Work out the finished part from the listing and answer in its coordinate system (mm). Face numbers are marked on the shaded views. A direction names the side the tool comes from. Round coordinates to 2 decimals unless told otherwise and drop trailing zeros. Loops run counter-clockwise (first coordinate to the right, second up) from the corner with the lowest first, then second, coordinate; pieces in that order, holes last.
```python
from build123d import *

# Parameters (mm, degrees)
SKETCH_W             = 28
SKETCH_H             = 22
PAD002_DEPTH         = 5
POCKET001_DEPTH      = 0.8
SKETCH002_W          = 0.6
SKETCH002_H          = 23
POCKET_DEPTH         = 4
LINEARPATTERN_COUNT  = 11
LINEARPATTERN_PITCH  = 1.9
POCKET002_DEPTH      = 3.5
SKETCH006_W          = 28
SKETCH006_H          = 22
POCKET005_DEPTH      = 1
POCKET005_DEPTH_BACK = 1
PAD_DEPTH            = 2


with BuildPart() as part:
    # Sketch → Pad002 (new body)
    with BuildSketch(Plane.XY):
        with Locations((15, 12)):
            Rectangle(SKETCH_W, SKETCH_H)
    extrude(amount=PAD002_DEPTH)

    # Sketch001 → Pocket001 (cut)
    with BuildSketch(Plane.XY):
        with BuildLine():
            ThreePointArc((17.967868, 19.714572), (14.962963, 20.499886), (11.967982, 19.677535))
            Line((11.967982, 19.677535), (4.036475, 13.531422))
            ThreePointArc((4.036475, 13.531422), (3.750333, 12.536475), (4, 11.531754))
            Line((4, 11.531754), (12.33, 4.876817))
            ThreePointArc((12.33, 4.876817), (15.374304, 4.261687), (18.318313, 5.25112))
            Line((18.318313, 5.25112), (26, 11.531754))
            ThreePointArc((26, 11.531754), (26.249667, 12.536475), (25.963525, 13.531422))
            Line((25.963525, 13.531422), (17.967868, 19.714572))
        make_face()
    extrude(amount=POCKET001_DEPTH, mode=Mode.SUBTRACT)

    # Sketch002 → Pocket (cut)
    with BuildSketch(Plane.XY):
        with Locations((6.3, 11.5)):
            Rectangle(SKETCH002_W, SKETCH002_H)
    pocket = extrude(amount=POCKET_DEPTH, mode=Mode.SUBTRACT)

    # LinearPattern: Pocket ×11
    with Locations(*[(i * LINEARPATTERN_PITCH, 0, 0) for i in range(1, LINEARPATTERN_COUNT)]):
        add(pocket, mode=Mode.SUBTRACT)

    # Sketch003 → Pocket002 (cut)
    with BuildSketch(Plane(origin=(0.5, 0, 4), x_dir=(0.707107, 0, -0.707107), z_dir=(0.707107, 0, 0.707107))):
        with BuildLine():
            ThreePointArc((17.966363, 19.215428), (14.961232, 19.999875), (11.966488, 19.17666))
            Line((11.966488, 19.17666), (4.036475, 13.531422))
            ThreePointArc((4.036475, 13.531422), (3.750333, 12.536475), (4, 11.531754))
            Line((4, 11.531754), (12.33, 5.376817))
            ThreePointArc((12.33, 5.376817), (15.374304, 4.761687), (18.318313, 5.75112))
            Line((18.318313, 5.75112), (26, 11.531754))
            ThreePointArc((26, 11.531754), (26.249667, 12.536475), (25.963525, 13.531422))
            Line((25.963525, 13.531422), (17.966363, 19.215428))
        make_face()
    extrude(amount=POCKET002_DEPTH, mode=Mode.SUBTRACT)

    # Sketch006 → Pocket005 (cut, two sides)
    with BuildSketch(Plane.XY.offset(5)) as pocket005_sk:
        with Locations((15, 12)):
            Rectangle(SKETCH006_W, SKETCH006_H)
        with BuildLine():
            ThreePointArc((17.966363, 19.215428), (14.961232, 19.999875), (11.966488, 19.17666))
            Line((11.966488, 19.17666), (4.036475, 13.531422))
            ThreePointArc((4.036475, 13.531422), (3.750333, 12.536475), (4, 11.531754))
            Line((4, 11.531754), (12.33, 5.376817))
            ThreePointArc((12.33, 5.376817), (15.374304, 4.761687), (18.318313, 5.75112))
            Line((18.318313, 5.75112), (26, 11.531754))
            ThreePointArc((26, 11.531754), (26.249667, 12.536475), (25.963525, 13.531422))
            Line((25.963525, 13.531422), (17.966363, 19.215428))
        make_face(mode=Mode.SUBTRACT)
    extrude(amount=-POCKET005_DEPTH, mode=Mode.SUBTRACT)
    extrude(pocket005_sk.sketch, amount=POCKET005_DEPTH_BACK, mode=Mode.SUBTRACT)

    # Sketch004 → Pad (join)
    with BuildSketch(Plane.XY.offset(5)):
        Polygon((5, 19.805), (25, 19.805), (25, 15), (30, 15), (30, 10), (25, 10), (25, 4.805), (5, 4.805), (5, 10), (0, 10), (0, 15), (5, 15), align=None)
    extrude(amount=PAD_DEPTH)


solid = part.part
```
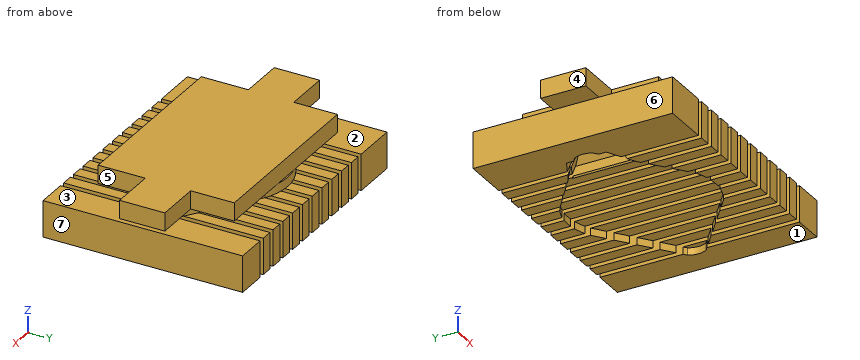
1. Find section A-A (x = 27). Write down the section's boundary in (y, z), then the cut area to 3 significant figures.
Answer key:
outline: (1, 0) - (23, 0) - (23, 4) - (1, 4) - close; (10, 5) - (15, 5) - (15, 7) - (10, 7) - close
area: 98.0 mm2
2. Find section D-D (x = 7). Write down the section's boundary in (y, z) (3 decimals), then the cut area to 3 significant figures.
Answer key:
outline: (1, 0) - (9.001, 0) - (9.135, 0.256) - (9.135, 0.8) - (9.419, 0.8) - (10.281, 2.45) - (14.71, 2.45) - (15.541, 0.8) - (15.828, 0.8) - (15.828, 0.23) - (15.943, 0) - (23, 0) - (23, 4) - (15.641, 4) - (15.641, 5) - (19.805, 5) - (19.805, 7) - (4.805, 7) - (4.805, 5) - (9.315, 5) - (9.315, 4) - (1, 4) - close
area: 110 mm2
3. Given pin 1 (3 mm diameter, centred on y = 13.5, z = 2, fed in from +X); pin 2 (0.7 mm diameter, centred on x = 14, y = 9, fed in from -Z); pin 3 (0.6 mm diameter, centred on x = 22.5, y = 20.5, fed in from +Z), each flat-ended and moving along its own axis, determine where each tip first touches the part or whether it passes through.
Answer key:
pin 1: stops at x = 29
pin 2: stops at z = 0.8
pin 3: stops at z = 4
4. Find section C-C (y = 3). Give the number of separate pieces and of enclosed holes in the cut face, then the cut area to 3 significant figures.
Answer key:
separate pieces: 12
enclosed holes: 0
area: 85.6 mm2
5. Consider probe 1 along Z at (x, y) = (11, 5.25); probe 2 along X at (y, z) = (11, 0.5); probe 3 along Z at (x, y) = (5.25, 21). Determine where each line is inside the solid, lowest interval first.
Answer key:
probe 1: z = 0 to 4, 5 to 7
probe 2: x = 1 to 4, 25.6 to 29
probe 3: z = 0 to 4
6. Determine the mould class of the marked faces 1, 2, 3 and 4 for opening direction Z: +Z half, -Z half, draft (parallel to the pull), parting line (faces both ways), or undercut.
Answer key:
face 1: -Z half
face 2: undercut
face 3: undercut
face 4: draft
7. Which of the six approach directions +Z, -Z, +X, -X, +Y, -Y give full straight-line access (tool end or side, diameter ignored) to the marked faces 5, 6 and 7?
Answer key:
face 5: +Z, -Z, +X, -Y
face 6: -Z, -X, +Y, -Y
face 7: -Z, +X, +Y, -Y
8. Find section B-B (z = 5.5). Write down the section's boundary in (x, y) (3 decimals), then the cut area to 3 significant figures.
Answer key:
outline: (0, 10) - (5, 10) - (5, 4.805) - (25, 4.805) - (25, 10) - (30, 10) - (30, 15) - (25, 15) - (25, 19.805) - (5, 19.805) - (5, 15) - (0, 15) - close
area: 350 mm2
